Could you check a few things on this model? Use its own coordinates, in mm. Face numbers are marked on the shaded views. A direction names the side the tool comes from. Give positions to 0.01 mm unless a question says otherwise; leave off trailing zeros. Loops run counter-clockwise (first coordinate to the right, second up) from the corner with the lowest first, then second, coordinate; pieces in that order, holes last. Notation, with made-up numbers: (15.5, 26) - (32.5, 26) arc R13 cw to (32.5, 48) - close; hole circle Ø3 at (-14, 55.25). An arc over 180 degrees is marked (long way). Write each question's results on one line, items separated by ' | '. Start each with the question number.
1) If we mould it in two halves opening along X, with no side actions, what happens to the marked faces 4, 5 and 6? For each: +X half, -X half, draft (parallel to the pull), parting line (faces both ways), or undercut.
2) On a 3-axis mill with a long thin cutter (end or side, diameter ignored), from which of +Z, -Z, +X, -X, +Y, -Y can I reach the whole of each face in a straight line? I mean the marked faces 1, 2 and 3. Say none if no direction works.
3) I want a section at B-B, the plane z = -6.25. Write out the boundary of the cut face in (x, y), and give its area (3 significant figures).
4) I'm going to push flat-ended pins straight in: pin 1 (5 mm diameter, centred on x = 21, z = -5.5, fed in from -Y); pin 2 (1.5 mm diameter, centred on x = 29, y = -3, fed in from -Z); pin 3 (5.5 mm diameter, centred on x = 1.5, y = 6.5, fed in from +Z); pin 4 (9 mm diameter, centred on x = -18, z = 0, fed in from +Y). Where does each tip first touch, or does it pass through?
5) If I drill on probe 1 along X at (y, z) = (-21, -0.5); probe 2 along X at (y, z) = (14, 7.75); probe 3 along Z at (x, y) = (-18, -7), over which ranges is the centre line in solid material (lowest first)? Write a range as [from, to].
6) I want a section at A-A, the plane x = -18. Write out the boundary of the cut face in (y, z), and give its area (3 significant figures).
7) I want a section at D-D, the plane z = 1. Write out the boundary of the cut face in (x, y).
8) I want a section at C-C, the plane y = 0. Write out the boundary of the cut face in (x, z).
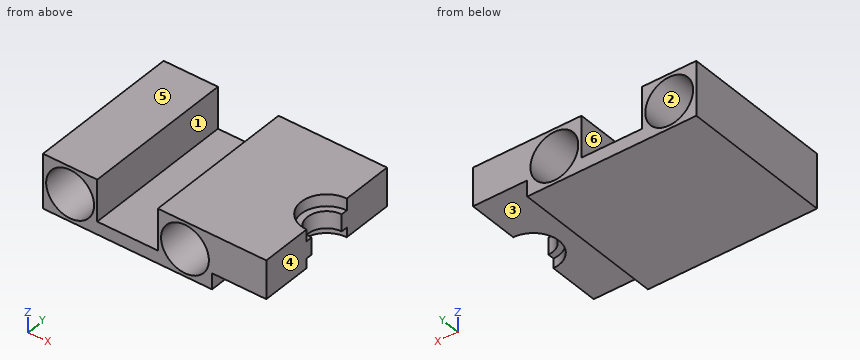
from build123d import *

# Parameters (mm, degrees)
SKETCH_R        = 7.5
PAD_DEPTH       = 24
SKETCH001_W     = 12
SKETCH001_H     = 48
PAD001_DEPTH    = 17
POCKET_DEPTH    = 17.001
POCKET001_DEPTH = 3.7
POCKET002_DEPTH = 3


with BuildPart() as part:
    # Sketch → Pad (new body, symmetric)
    with BuildSketch(Plane.XZ):
        Polygon((-26.5, 8.5), (-26.5, -8.5), (26.5, -8.5), (26.5, 8.5), (9.5, 8.5), (9.5, -4.5), (-9.5, -4.5), (-9.5, 8.5), align=None)
        with Locations((-18, 0)):
            Circle(SKETCH_R, mode=Mode.SUBTRACT)
        with Locations((18, 0)):
            Circle(SKETCH_R, mode=Mode.SUBTRACT)
    extrude(amount=PAD_DEPTH, both=True)

    # Sketch001 → Pad001 (new body)
    with BuildSketch(Plane(origin=(26.5, 0, 0), x_dir=(0, 0, 1), z_dir=(1, 0, 0))):
        with Locations((2.5, 0)):
            Rectangle(SKETCH001_W, SKETCH001_H)
    extrude(amount=PAD001_DEPTH)

    # Sketch002 → Pocket (cut, through all)
    with BuildSketch(Plane(origin=(0, 0, 8.5), x_dir=(-1, 0, 0), z_dir=(0, 0, 1))):
        with BuildLine():
            ThreePointArc((-43.5, -6), (-37.5, 0), (-43.5, 6))
            Line((-43.5, 6), (-55.5, 6))
            Line((-55.5, 6), (-55.5, -6))
            Line((-55.5, -6), (-43.5, -6))
        make_face()
    extrude(amount=-POCKET_DEPTH, mode=Mode.SUBTRACT)

    # Sketch003 → Pocket001 (cut)
    with BuildSketch(Plane(origin=(0, 0, 8.5), x_dir=(-1, 0, 0), z_dir=(0, 0, 1))):
        with BuildLine():
            ThreePointArc((-43.50003, -8), (-35.5, -1.5e-05), (-43.5, 8))
            Line((-43.5, 8), (-59.5, 8))
            Line((-59.5, 8), (-59.5, -8))
            Line((-59.5, -8), (-43.50003, -8))
        make_face()
    extrude(amount=-POCKET001_DEPTH, mode=Mode.SUBTRACT)

    # Sketch004 → Pocket002 (cut)
    with BuildSketch(Plane(origin=(0, 0, -3.5), x_dir=(1, 0, 0), z_dir=(0, 0, -1))):
        with BuildLine():
            ThreePointArc((43.5, 8), (35.500027, -1.3e-05), (43.500027, -8))
            Line((59.500053, -8), (43.500027, -8))
            Line((59.500053, 8.000053), (59.500053, -8))
            Line((43.5, 8), (59.500053, 8.000053))
        make_face()
    extrude(amount=-POCKET002_DEPTH, mode=Mode.SUBTRACT)


solid = part.part
Answers:
1) face 4: +X half | face 5: draft | face 6: undercut
2) face 1: +Z, +Y, -Y | face 2: +Y, -Y | face 3: -Z, +X, +Y, -Y
3) outline: (-26.5, -24) - (-22.15, -24) - (-22.15, 24) - (-26.5, 24) - close; (-13.85, -24) - (13.85, -24) - (13.85, 24) - (-13.85, 24) - close; (22.15, -24) - (26.5, -24) - (26.5, 24) - (22.15, 24) - close | area: 1,750 mm2
4) pin 1: stops at y = -24 | pin 2: stops at z = -3.5 | pin 3: stops at z = -4.5 | pin 4: passes through
5) probe 1: x = [-26.5, -25.48], [-10.52, -9.5], [9.5, 10.52], [25.48, 43.5] | probe 2: x = [-26.5, -9.5], [9.5, 43.5] | probe 3: z = [-8.5, -7.5], [7.5, 8.5]
6) outline: (-24, -8.5) - (24, -8.5) - (24, -7.5) - (-24, -7.5) - close; (-24, 7.5) - (24, 7.5) - (24, 8.5) - (-24, 8.5) - close | area: 96.0 mm2
7) outline: (-26.5, -24) - (-25.43, -24) - (-25.43, 24) - (-26.5, 24) - close; (-10.57, -24) - (-9.5, -24) - (-9.5, 24) - (-10.57, 24) - close; (9.5, -24) - (10.57, -24) - (10.57, 24) - (9.5, 24) - close; (25.43, -24) - (43.5, -24) - (43.5, -6) arc R6 cw to (43.5, 6) - (43.5, 24) - (25.43, 24) - close
8) outline: (-26.5, -8.5) - (26.5, -8.5) - (26.5, -3.5) - (35.5, -3.5) - (35.5, -0.5) - (37.5, -0.5) - (37.5, 4.8) - (35.5, 4.8) - (35.5, 8.5) - (9.5, 8.5) - (9.5, -4.5) - (-9.5, -4.5) - (-9.5, 8.5) - (-26.5, 8.5) - close; hole circle Ø15 at (-18, 0); hole circle Ø15 at (18, 0)
